```python
from build123d import *

# Parameters (mm, degrees)
F1_DEPTH = 6.35
F3_DEPTH = 12.7
F5_DEPTH = 6.35
F6_R     = 5.08
F7_R     = 5.08
F8_R     = 5.08


with BuildPart() as f1:
    # F0 (on Front) → F1 (new body)
    with BuildSketch(Plane.XZ):
        with BuildLine():
            Line((-29.225341, 25.4), (-38.1, 25.4))
            Line((-38.1, 25.4), (-38.1, 0))
            Line((-38.1, 0), (-30.507866, 0))
            ThreePointArc((-30.507866, 0), (-20.531018, 9.976848), (-10.554171, 0))
            Line((-10.554171, 0), (11.91838, 0))
            ThreePointArc((11.91838, 0), (21.895228, 9.976848), (31.872075, 0))
            Line((31.872075, 0), (38.1, 0))
            Line((38.1, 0), (38.1, 19.05))
            Line((38.1, 19.05), (22.325266, 19.05))
            Line((22.325266, 19.05), (9.537391, 33.169942))
            Line((9.537391, 33.169942), (-9.512609, 33.169942))
            Line((-9.512609, 33.169942), (-9.512609, 19.05))
            Line((-9.512609, 19.05), (-29.225341, 19.05))
            Line((-29.225341, 19.05), (-29.225341, 25.4))
        make_face()
    extrude(amount=F1_DEPTH)

    # F2 (on face) → F3 (join)
    with BuildSketch(Plane.XZ.offset(6.35)):
        with BuildLine():
            Line((-29.225341, 25.4), (-38.1, 25.4))
            Line((-38.1, 25.4), (-38.1, 0))
            Line((-38.1, 0), (-22.118518, 0))
            ThreePointArc((-22.118518, 0), (-20.531018, 1.5875), (-18.943518, 0))
            Line((-18.943518, 0), (20.268538, 0))
            ThreePointArc((20.268538, 0), (21.856038, 1.5875), (23.443538, 0))
            Line((23.443538, 0), (38.1, 0))
            Line((38.1, 0), (38.1, 19.05))
            Line((38.1, 19.05), (22.325266, 19.05))
            Line((22.325266, 19.05), (9.537391, 33.169942))
            Line((9.537391, 33.169942), (-9.512609, 33.169942))
            Line((-9.512609, 33.169942), (-9.512609, 19.05))
            Line((-9.512609, 19.05), (-29.225341, 19.05))
            Line((-29.225341, 19.05), (-29.225341, 25.4))
        make_face()
        with BuildLine():
            Line((-22.118518, 0), (-38.1, 0))
            Line((-38.1, 0), (-38.1, -4.83568))
            Line((-38.1, -4.83568), (38.1, -4.83568))
            Line((38.1, -4.83568), (38.1, 0))
            Line((38.1, 0), (23.443538, 0))
            ThreePointArc((23.443538, 0), (21.856038, -1.5875), (20.268538, 0))
            Line((20.268538, 0), (-18.943518, 0))
            ThreePointArc((-18.943518, 0), (-20.531018, -1.5875), (-22.118518, 0))
        make_face()
    extrude(amount=F3_DEPTH)

    # F4 (on face) → F5 (join)
    with BuildSketch(Plane.XZ.offset(19.05)):
        with BuildLine():
            Line((-29.225341, 25.4), (-38.1, 25.4))
            Line((-38.1, 25.4), (-38.1, 0))
            Line((-38.1, 0), (-30.507866, 0))
            ThreePointArc((-30.507866, 0), (-20.531018, 9.976848), (-10.554171, 0))
            Line((-10.554171, 0), (11.91838, 0))
            ThreePointArc((11.91838, 0), (21.895228, 9.976848), (31.872075, 0))
            Line((31.872075, 0), (38.1, 0))
            Line((38.1, 0), (38.1, 19.05))
            Line((38.1, 19.05), (22.325266, 19.05))
            Line((22.325266, 19.05), (9.537391, 33.169942))
            Line((9.537391, 33.169942), (-9.512609, 33.169942))
            Line((-9.512609, 33.169942), (-9.512609, 19.05))
            Line((-9.512609, 19.05), (-29.225341, 19.05))
            Line((-29.225341, 19.05), (-29.225341, 25.4))
        make_face()
    extrude(amount=F5_DEPTH)

    # F6
    f6_edges = [f1.edges().sort_by_distance(p)[0] for p in [
        (-29.225341, -12.7, 25.4),
    ]]
    fillet(f6_edges, radius=F6_R)

    # F7
    f7_edges = [f1.edges().sort_by_distance(p)[0] for p in [
        (9.537391, -12.7, 33.169942),
    ]]
    fillet(f7_edges, radius=F7_R)

    # F8
    f8_edges = [f1.edges().sort_by_distance(p)[0] for p in [
        (22.325266, -12.7, 19.05),
        (38.1, -12.7, 19.05),
    ]]
    fillet(f8_edges, radius=F8_R)


solid = f1.part
```
Model file for the job. Use its own axes, mm. A direction names the side the tool comes from. Give positions to 0.01 mm unless a question says otherwise; leave off trailing zeros. Order: outer loops, then holes, each group sorted by start corner. A loop starts at its lowest first (then second) coordinate and runs counter-clockwise, first axis right, second up.
1) Mould opens along X. For faces 1 (the flat face through (-38.1, -13, 10)), 2 (the flat face through (-9.513, -13, 26)), 3 (the flat face through (1, -22, 0)), 4 (the flat face through (-1, -19.05, -1)) say: +X half, -X half, draft (parallel to the pull), parting line (faces both ways), or undercut.
2) Wall check: probe 1 along X at (y, z) = (-9.5, 0); probe 2 along Y at (x, z) = (4, -2); probe 3 along Z at (x, y) = (-16, -16). Give the ranges that are in metal, low to high.
3) Pin check, flat tips, straight feed: pin 1 (3 mm diameter, centred on x = -36, y = -10, fed in from +Z); pin 2 (5 mm diameter, centred on x = -0.5, y = -22, fed in from -Z); pin 3 (3.5 mm diameter, centred on x = 21.86, z = 0, fed in from -Y); pin 4 (2.5 mm diameter, centred on x = -20.53, z = 0, fed in from -Y). Stop position of each tip, or through.
4) Saw through at A-A, the plane y = -9.25. Count the separate pieces of the cut face and the enclosed holes in it, then the cut area to 3 significant figures.
5) 3-axis set-ups, long thin cutter, end or side, ignore diameter. For faces 5 (the flat face through (-36, -13, 25.4)), 6 (the flat face through (1, -3, 0)), 7 (the flat face through (29, -13, 19.05)): which of +Z, -Z, +X, -X, +Y, -Y reach the whole face in a straight line?
6) Saw through at B-B, the plane z = 23. Write the cut outline in (x, y).
7) Saw through at C-C, the plane y = -22.75. Write the cut outline in (x, z).
8) Saw through at D-D, the plane x = -15. Write the cut outline in (y, z).
Computed:
1. face 1: -X half
1. face 2: undercut
1. face 3: draft
1. face 4: undercut
2. probe 1: x = -38.1 to -22.12, -18.94 to 20.27, 23.44 to 38.1
2. probe 2: y = -19.05 to -6.35
2. probe 3: z = -4.84 to 19.05
3. pin 1: stops at z = 25.4
3. pin 2: stops at z = 0
3. pin 3: stops at y = -19.05
3. pin 4: passes through
4. separate pieces: 1
4. enclosed holes: 2
4. area: 2,210 mm2
5. face 5: +Z, -X, +Y, -Y
5. face 6: -Z, +X, -X, +Y
5. face 7: +Z, +X, +Y, -Y
6. outline: (-38.1, -25.4) - (-29.99, -25.4) - (-29.99, 0) - (-38.1, 0) - close; (-9.51, -25.4) - (18.75, -25.4) - (18.75, 0) - (-9.51, 0) - close
7. outline: (-38.1, 0) - (-30.51, 0) arc R9.98 cw to (-10.55, 0) - (11.92, 0) arc R9.98 cw to (31.87, 0) - (38.1, 0) - (38.1, 13.97) arc R5.08 ccw to (33.02, 19.05) - (24.58, 19.05) arc R5.08 cw to (20.81, 20.72) - (11.05, 31.5) arc R5.08 ccw to (7.28, 33.17) - (-9.51, 33.17) - (-9.51, 19.05) - (-29.23, 19.05) - (-29.23, 20.32) arc R5.08 ccw to (-34.31, 25.4) - (-38.1, 25.4) - close
8. outline: (-25.4, 8.3) - (-19.05, 8.3) - (-19.05, -4.84) - (-6.35, -4.84) - (-6.35, 8.3) - (0, 8.3) - (0, 19.05) - (-25.4, 19.05) - close
